CAD build for the part. Positions are in the model's coordinates, mm. A direction names the side the tool comes from. Give positions to 0.01 mm unless a question says otherwise; leave off trailing zeros. Write each loop counter-clockwise with the first axis right and the second up, starting at its lowest first coordinate (ties: lowest second). Pieces come first, ordered by that corner, then holes. Notation, with made-up numbers: (-23, 25.25) -> (-13, 25.25) arc R23 ccw to (-13, 40.25) -> close; hole circle Ø7 at (70, 6.5). An arc over 180 degrees is marked (long way). Answer in a Markdown table with one row per item. Add a question column.
```python
from build123d import *

# Parameters (mm, degrees)
BOSS_EXTRU_1_DEPTH      = 0.7
ENL_V_MAT_EXTRU_1_DEPTH = 0.1
BOSS_EXTRU_2_START      = 0.7
BOSS_EXTRU_2_DEPTH      = 0.7
ESQUISSE4_R             = 3
BOSS_EXTRU_3_DEPTH      = 0.7
CONG_1_R                = 0.1
ESQUISSE5_R             = 2.9
BOSS_EXTRU_4_DEPTH      = 0.5
ESQUISSE6_R             = 3
BOSS_EXTRU_5_DEPTH      = 3.7
CONG_2_R                = 0.4
CONG_3_R                = 0.3
ESQUISSE7_W             = 1.2
ESQUISSE7_H             = 0.1
BOSS_EXTRU_6_DEPTH      = 0.8
CONG_4_R                = 0.1
CONG_5_R                = 0.1
ESQUISSE8_W             = 1.2
ESQUISSE8_H             = 0.1
BOSS_EXTRU_7_DEPTH      = 0.8
CONG_6_R                = 0.1
CONG_7_R                = 0.1


with BuildPart() as part:
    # Esquisse1 → Boss.-Extru.1 (new body)
    with BuildSketch(Plane(origin=(0, 0, 0), x_dir=(1, 0, 0), z_dir=(0, 1, 0))):
        Polygon((4.959009742, 6.55), (6.55, 4.959009742), (6.55, 1.590990258), (4.959009742, 0), (0, 0), (0, 6.55), align=None)
    extrude(amount=BOSS_EXTRU_1_DEPTH)

    # Esquisse2 → Enlèv. mat.-Extru.1 (cut)
    with BuildSketch(Plane(origin=(0, 0.7, 0), x_dir=(1, 0, 0), z_dir=(0, 1, 0))):
        with BuildLine():
            Line((2.275, 6.55), (4.275, 6.55))
            Line((4.275, 6.55), (4.275, 6.156405907))
            ThreePointArc((4.275, 6.156405907), (5.431675683, 5.431675683), (6.156405907, 4.275))
            Line((6.156405907, 4.275), (6.55, 4.275))
            Line((6.55, 4.275), (6.55, 2.275))
            Line((6.55, 2.275), (6.156405907, 2.275))
            ThreePointArc((6.156405907, 2.275), (5.431675683, 1.118324317), (4.275, 0.393594093))
            Line((4.275, 0.393594093), (4.275, 0))
            Line((4.275, 0), (2.275, 0))
            Line((2.275, 0), (2.275, 0.393594093))
            ThreePointArc((2.275, 0.393594093), (1.118324317, 1.118324317), (0.393594093, 2.275))
            Line((0.393594093, 2.275), (0, 2.275))
            Line((0, 2.275), (0, 4.275))
            Line((0, 4.275), (0.393594093, 4.275))
            ThreePointArc((0.393594093, 4.275), (1.118324317, 5.431675683), (2.275, 6.156405907))
            Line((2.275, 6.156405907), (2.275, 6.55))
        make_face()
    extrude(amount=-ENL_V_MAT_EXTRU_1_DEPTH, mode=Mode.SUBTRACT)

    # Esquisse3 → Boss.-Extru.2 (add)
    with BuildSketch(Plane(origin=(0, 0.7, 0), x_dir=(1, 0, 0), z_dir=(0, 1, 0)).offset(BOSS_EXTRU_2_START)):
        with BuildLine():
            Line((0, 0), (2.275, 0))
            Line((2.275, 0), (2.275, 0.393594093))
            ThreePointArc((2.275, 0.393594093), (1.118324317, 1.118324317), (0.393594093, 2.275))
            Line((0.393594093, 2.275), (0, 2.275))
            Line((0, 2.275), (0, 0))
        make_face()
        with BuildLine():
            Line((0, 6.55), (0, 4.275))
            Line((0, 4.275), (0.393594093, 4.275))
            ThreePointArc((0.393594093, 4.275), (1.118324317, 5.431675683), (2.275, 6.156405907))
            Line((2.275, 6.156405907), (2.275, 6.55))
            Line((2.275, 6.55), (0, 6.55))
        make_face()
    extrude(amount=-BOSS_EXTRU_2_DEPTH)

    # Esquisse4 → Boss.-Extru.3 (add)
    with BuildSketch(Plane(origin=(0, 0.6, 0), x_dir=(1, 0, 0), z_dir=(0, 1, 0))):
        with Locations(Location((3.275, 3.275, 0), (0, 0, 270))):
            Circle(ESQUISSE4_R)
    extrude(amount=BOSS_EXTRU_3_DEPTH)

    # Congé1
    cong_1_edges = [part.edges().sort_by_distance(p)[0] for p in [
        (3.275, 1.3, -6.275),
    ]]
    fillet(cong_1_edges, radius=CONG_1_R)

    # Esquisse5 → Boss.-Extru.4 (add)
    with BuildSketch(Plane(origin=(0, 1.3, 0), x_dir=(1, 0, 0), z_dir=(0, 1, 0))):
        with Locations(Location((3.275, 3.275, 0), (0, 0, 270))):
            Circle(ESQUISSE5_R)
    extrude(amount=BOSS_EXTRU_4_DEPTH)

    # Esquisse6 → Boss.-Extru.5 (add)
    with BuildSketch(Plane(origin=(0, 1.8, 0), x_dir=(1, 0, 0), z_dir=(0, 1, 0))):
        with Locations(Location((3.275, 3.275, 0), (0, 0, 270))):
            Circle(ESQUISSE6_R)
    extrude(amount=BOSS_EXTRU_5_DEPTH)

    # Congé2
    # the kernel refuses this fillet: 0.4 mm, written as the material it takes off along each edge
    with BuildSketch(Plane(origin=(3.275, 1.8, -3.275), x_dir=(0, 0, 1), z_dir=(-1, 0, 0))) as cong_2_piece_1:
        with BuildLine():
            CenterArc((2.6, 0.264575131), CONG_2_R, 318.590377891, 41.409622109)
            Line((2.9, 0), (2.906, -0.005291503))
            ThreePointArc((2.906, -0.005291503), (2.95, -0.008), (3, -0.008))
            Line((3, -0.008), (3.008, 0))
            Line((3.008, 0), (3.008, 0.264575131))
            Line((3.008, 0.264575131), (3, 0.264575131))
        make_face()
    revolve(axis=Axis((3.275, 1.8, -3.275), (0, 1, 0)), mode=Mode.SUBTRACT)

    # Congé3
    cong_3_edges = [part.edges().sort_by_distance(p)[0] for p in [
        (3.275, 5.5, -6.275),
    ]]
    fillet(cong_3_edges, radius=CONG_3_R)

    # Esquisse7 → Boss.-Extru.6 (add)
    with BuildSketch(Plane(origin=(6.55, 0, 0), x_dir=(0, 0, -1), z_dir=(1, 0, 0))):
        with Locations((3.275, 0.05)):
            Rectangle(ESQUISSE7_W, ESQUISSE7_H)
    extrude(amount=BOSS_EXTRU_6_DEPTH)

    # Congé4
    cong_4_edges = [part.edges().sort_by_distance(p)[0] for p in [
        (6.55, 0.1, -3.275),
    ]]
    fillet(cong_4_edges, radius=CONG_4_R)

    # Congé5
    # the kernel refuses this fillet: 0.1 mm, written as the material it takes off along each edge
    with BuildSketch(Plane(origin=(6.65, 0.2, -3.875), x_dir=(0.8017442392976484, 0.5976672776328275, 0), z_dir=(0.5976672776328275, -0.8017442392976484, 0))) as cong_5_piece_1_section:
        with BuildLine():
            CenterArc((0.1 + CONG_5_R, CONG_5_R), CONG_5_R, 180, 90)
            Line((0.1 + CONG_5_R, 0), (0.1, 0))
            Line((0.1, 0), (0.1, CONG_5_R))
        make_face()
    cong_5_piece_1 = revolve(axis=Axis((6.65, 0.2, -3.875), (0, 0, 1)), revolution_arc=233.296989237, mode=Mode.PRIVATE)
    cong_5_piece_1 = split(cong_5_piece_1, bisect_by=Plane(origin=(6.55, 0.125006103, -3.843837174), z_dir=(1, 0, 0)), keep=Keep.TOP, mode=Mode.PRIVATE)
    add(cong_5_piece_1, mode=Mode.SUBTRACT)
    with BuildSketch(Plane(origin=(6.65, 0.2, -2.675), x_dir=(0.8017442392976484, 0.5976672776328275, 0), z_dir=(0.5976672776328275, -0.8017442392976484, 0))) as cong_5_piece_2_section:
        with BuildLine():
            CenterArc((0.1 + CONG_5_R, -CONG_5_R), CONG_5_R, 90, 90)
            Line((0.1 + CONG_5_R, 0), (0.1, 0))
            Line((0.1, 0), (0.1, -CONG_5_R))
        make_face()
    cong_5_piece_2 = revolve(axis=Axis((6.65, 0.2, -2.675), (0, 0, 1)), revolution_arc=233.296989237, mode=Mode.PRIVATE)
    cong_5_piece_2 = split(cong_5_piece_2, bisect_by=Plane(origin=(6.55, 0.125006105, -2.706162828), z_dir=(1, 0, 0)), keep=Keep.TOP, mode=Mode.PRIVATE)
    add(cong_5_piece_2, mode=Mode.SUBTRACT)
    with BuildSketch(Plane(origin=(7.35, 0.1, -4.125), x_dir=(-1, 0, 0), z_dir=(0, 0, 1))) as cong_5_piece_3:
        with BuildLine():
            CenterArc((CONG_5_R, CONG_5_R), CONG_5_R, 180, 90)
            Line((0, CONG_5_R), (0, 0))
            Line((0, 0), (CONG_5_R, 0))
        make_face()
    extrude(amount=1.7, mode=Mode.SUBTRACT)
    with BuildSketch(Plane(origin=(6.65, 0.1, -3.875), x_dir=(0, 0, 1), z_dir=(1, 0, 0))) as cong_5_piece_4:
        with BuildLine():
            CenterArc((CONG_5_R, CONG_5_R), CONG_5_R, 180, 90)
            Line((0, CONG_5_R), (0, 0))
            Line((0, 0), (CONG_5_R, 0))
        make_face()
    extrude(amount=0.95, mode=Mode.SUBTRACT)
    with BuildSketch(Plane(origin=(6.65, 0.1, -2.675), x_dir=(0, 0, -1), z_dir=(1, 0, 0))) as cong_5_piece_5:
        with BuildLine():
            CenterArc((CONG_5_R, -CONG_5_R), CONG_5_R, 90, 90)
            Line((0, -CONG_5_R), (0, 0))
            Line((0, 0), (CONG_5_R, 0))
        make_face()
    extrude(amount=0.95, mode=Mode.SUBTRACT)

    # Esquisse8 → Boss.-Extru.7 (add)
    with BuildSketch(Plane.ZY):
        with Locations((-3.275, 0.05)):
            Rectangle(ESQUISSE8_W, ESQUISSE8_H)
    extrude(amount=BOSS_EXTRU_7_DEPTH)

    # Congé6
    cong_6_edges = [part.edges().sort_by_distance(p)[0] for p in [
        (0, 0.1, -3.275),
    ]]
    fillet(cong_6_edges, radius=CONG_6_R)

    # Congé7
    # the kernel refuses this fillet: 0.1 mm, written as the material it takes off along each edge
    with BuildSketch(Plane(origin=(-0.1, 0.2, -2.675), x_dir=(-0.8017442392976492, 0.5976672776328262, 0), z_dir=(-0.5976672776328262, -0.8017442392976492, 0))) as cong_7_piece_1_section:
        with BuildLine():
            CenterArc((0.1 + CONG_7_R, CONG_7_R), CONG_7_R, 180, 90)
            Line((0.1, CONG_7_R), (0.1, 0))
            Line((0.1, 0), (0.1 + CONG_7_R, 0))
        make_face()
    cong_7_piece_1 = revolve(axis=Axis((-0.1, 0.2, -2.675), (0, 0, -1)), revolution_arc=233.296989237, mode=Mode.PRIVATE)
    cong_7_piece_1 = split(cong_7_piece_1, bisect_by=Plane(origin=(0, 0.125006101, -2.706162827), z_dir=(-1, 0, 0)), keep=Keep.TOP, mode=Mode.PRIVATE)
    add(cong_7_piece_1, mode=Mode.SUBTRACT)
    with BuildSketch(Plane(origin=(-0.1, 0.2, -3.875), x_dir=(-0.801744239297649, 0.5976672776328265, 0), z_dir=(-0.5976672776328265, -0.801744239297649, 0))) as cong_7_piece_2_section:
        with BuildLine():
            CenterArc((0.1 + CONG_7_R, -CONG_7_R), CONG_7_R, 90, 90)
            Line((0.1 + CONG_7_R, 0), (0.1, 0))
            Line((0.1, 0), (0.1, -CONG_7_R))
        make_face()
    cong_7_piece_2 = revolve(axis=Axis((-0.1, 0.2, -3.875), (0, 0, -1)), revolution_arc=233.296989237, mode=Mode.PRIVATE)
    cong_7_piece_2 = split(cong_7_piece_2, bisect_by=Plane(origin=(0, 0.125006106, -3.843837173), z_dir=(-1, 0, 0)), keep=Keep.TOP, mode=Mode.PRIVATE)
    add(cong_7_piece_2, mode=Mode.SUBTRACT)
    with BuildSketch(Plane(origin=(-0.1, 0.1, -2.675), x_dir=(0, 0, -1), z_dir=(-1, 0, 0))) as cong_7_piece_3:
        with BuildLine():
            CenterArc((CONG_7_R, CONG_7_R), CONG_7_R, 180, 90)
            Line((0, CONG_7_R), (0, 0))
            Line((0, 0), (CONG_7_R, 0))
        make_face()
    extrude(amount=0.95, mode=Mode.SUBTRACT)
    with BuildSketch(Plane(origin=(-0.8, 0.1, -4.125), x_dir=(0, -1, 0), z_dir=(0, 0, 1))) as cong_7_piece_4:
        with BuildLine():
            CenterArc((CONG_7_R, CONG_7_R), CONG_7_R, 180, 90)
            Line((0, CONG_7_R), (0, 0))
            Line((0, 0), (CONG_7_R, 0))
        make_face()
    extrude(amount=1.7, mode=Mode.SUBTRACT)
    with BuildSketch(Plane(origin=(-0.1, 0.1, -3.875), x_dir=(0, 0, 1), z_dir=(-1, 0, 0))) as cong_7_piece_5:
        with BuildLine():
            CenterArc((CONG_7_R, -CONG_7_R), CONG_7_R, 90, 90)
            Line((0, -CONG_7_R), (0, 0))
            Line((0, 0), (CONG_7_R, 0))
        make_face()
    extrude(amount=0.95, mode=Mode.SUBTRACT)


solid = part.part
```
Item 1: Mould opens along Z. For faces 6 (the face through (0.346, 0.896, -3.925)), 7 (the face through (1, 1.4, -6)), 8 (the face through (5.74, 0.35, -5.77)) say: released by +Z, released by -Z, zero draft, split by the parting line, or undercut.
Item 2: Slice it at A-A, the plane y = 2.85. List the corners of the cut face in (x, z) (3 decimals).
Item 3: Which spindle directions (+Z, -Z, +X, -X, +Y, -Y) get a long thin tool onto all of the face, cutting with end or side? Do faces 1 (the face through (5.59, 0.7, -1.06)), 2 (the face through (0.444, 1.546, -3.904)), 3 (the face through (1, 1.4, -1)), 4 (the face through (2, 1, -6.55)), 5 (the face through (0.346, 3.61, -3.925)). Say none if no direction does.
Item 4: Probe L1, parallel to X at y = 4.2, z = -2.5; L2, parallel to Y at x = 3.25, z = -6; L3, parallel to Y at x = 0.25, z = -2. List the from-to ranges inside material, lowest first. Write a range as from..to.
Item 5: Drop flat-ended pins along their axis: pin 1 Ø2 at (x, y) = (4, 2) entering from +Z (3 decimals); pin 2 Ø1.5 at (y, z) = (5, -4) entering from -X (3 decimals). Give the stop position or say it passes through.
Answer key:
| question | item | result |
|---|---|---|
| 1 | face 6 | undercut |
| 1 | face 7 | zero draft |
| 1 | face 8 | released by -Z |
| 2 | outline | circle Ø6 at (3.275, -3.275) |
| 3 | face 1 | +Z, +X, +Y |
| 3 | face 2 | none |
| 3 | face 3 | +Z, -X, +Y |
| 3 | face 4 | -Z, +X, -X, +Y, -Y |
| 3 | face 5 | +Y |
| 4 | L1 | x = 0.38..6.17 |
| 4 | L2 | y = 0..5.5 |
| 4 | L3 | y = 0..1.4 |
| 5 | pin 1 | stops at z = -0.275 |
| 5 | pin 2 | stops at x = 0.275 |
